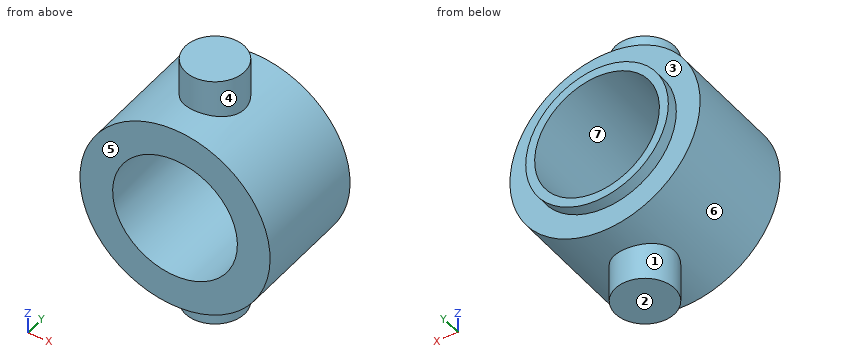
from build123d import *

# Parameters (mm, degrees)
SKETCH1_R           = 8
SKETCH1_R_2         = 5.25
BOSS_EXTRUDE1_DEPTH = 5
SKETCH2_R           = 6
SKETCH2_R_2         = 5.25
BOSS_EXTRUDE2_DEPTH = 1
SKETCH3_R           = 2.5
BOSS_EXTRUDE3_DEPTH = 5


with BuildPart() as part:
    # Sketch1 → Boss-Extrude1 (new, symmetric)
    with BuildSketch(Plane(origin=(0, 0, 0), x_dir=(1, 0, 0), z_dir=(0, 1, 0))):
        with Locations(Location((0, 0, 0), (0, 0, 270))):
            Circle(SKETCH1_R)
        with Locations(Location((0, 0, 0), (0, 0, 270))):
            Circle(SKETCH1_R_2, mode=Mode.SUBTRACT)
    extrude(amount=BOSS_EXTRUDE1_DEPTH, both=True)

    # Sketch2 → Boss-Extrude2 (add, symmetric)
    with BuildSketch(Plane(origin=(0, 5, 0), x_dir=(1, 0, 0), z_dir=(0, 1, 0))):
        with Locations(Location((0, 0, 0), (0, 0, 270))):
            Circle(SKETCH2_R)
        with Locations(Location((0, 0, 0), (0, 0, 270))):
            Circle(SKETCH2_R_2, mode=Mode.SUBTRACT)
    extrude(amount=BOSS_EXTRUDE2_DEPTH, both=True)

    # Sketch3 → Boss-Extrude3 (add)
    with BuildSketch(Plane.XY.offset(6)):
        with Locations(Location((0, 0, 0), (0, 0, 180))):
            Circle(SKETCH3_R)
    boss_extrude3 = extrude(amount=BOSS_EXTRUDE3_DEPTH)

    # Mirror1: Boss-Extrude3 across plane
    add(boss_extrude3.mirror(Plane.XY))


solid = part.part
Can you work these out from the model? Positions are in its coordinate system, mm. Face numbers are marked on the shaded views. A direction names the side the tool comes from. Coordinates: 2 decimals unless noted, no trailing zeros. Write each loop counter-clockwise with the first axis right and the second up, starting at its lowest first coordinate (ties: lowest second). Pieces come first, ordered by that corner, then holes. Notation, with made-up numbers: (-14, 14) -> (6, 14) arc R24 ccw to (6, 37) -> close; hole circle Ø5 at (-24.75, 81). An arc over 180 degrees is marked (long way). Write item = value, one per line.
(1) Imagine slicing it at D-D (x = 2.25). Please give me the cut outline in (y, z).
Verdict:
outline = (-5, -7.68) -> (-1.09, -7.68) -> (-1.09, -11) -> (1.09, -11) -> (1.09, -7.68) -> (5, -7.68) -> (5, -5.56) -> (6, -5.56) -> (6, -4.74) -> (-5, -4.74) -> close; (-5, 4.74) -> (6, 4.74) -> (6, 5.56) -> (5, 5.56) -> (5, 7.68) -> (1.09, 7.68) -> (1.09, 11) -> (-1.09, 11) -> (-1.09, 7.68) -> (-5, 7.68) -> close
(2) If I drill on probe 1 along X at (y, z) = (3.25, 0); probe 2 along Y at (x, z) = (-5, 4); probe 3 along Z at (x, y) = (-3, -4), over which ranges is the centre line in solid material (lowest first)?
Verdict:
probe_1 = -8 to -5.25, 5.25 to 8
probe_2 = -5 to 5
probe_3 = -7.42 to -4.31, 4.31 to 7.42
(3) Imagine slicing it at C-C (y = 0). Please give me the cut outline in (x, z).
Verdict:
outline = (-2.5, -11) -> (2.5, -11) -> (2.5, -7.6) arc R8 ccw to (2.5, 7.6) -> (2.5, 11) -> (-2.5, 11) -> (-2.5, 7.6) arc R8 ccw to (-2.5, -7.6) -> close; hole circle Ø10.5 at (0, 0)
(4) For pin 1 (2 mm diameter, centred on y = 0, z = 2, fed in from -X); pin 2 (5 mm diameter, centred on y = 3, z = -4, fed in from +X); pin 3 (4 mm diameter, centred on y = 1, z = -7.5, fed in from +X), each with a flat end and sliding along its axis, tell me the tip position at first contact or that it passes through.
Verdict:
pin_1 = -7.94
pin_2 = 7.86
pin_3 = 5.81
(5) Imagine slicing it at B-B (x = 0). Please give me the cut outline in (y, z), and give its area (3 significant figures).
Verdict:
outline = (-5, -8) -> (-2.5, -8) -> (-2.5, -11) -> (2.5, -11) -> (2.5, -8) -> (5, -8) -> (5, -6) -> (6, -6) -> (6, -5.25) -> (-5, -5.25) -> close; (-5, 5.25) -> (6, 5.25) -> (6, 6) -> (5, 6) -> (5, 8) -> (2.5, 8) -> (2.5, 11) -> (-2.5, 11) -> (-2.5, 8) -> (-5, 8) -> close
area = 86.5 mm^2
(6) On a 3-axis mill with a long thin cutter (end or side, diameter ignored), from which of +Z, -Z, +X, -X, +Y, -Y can I reach the whole of each face in a straight line? I mean the marked faces 1, 2, 3 and 4. Say none if no direction works.
Verdict:
face_1 = -Z
face_2 = -Z, +X, -X, +Y, -Y
face_3 = +Y
face_4 = +Z
(7) Thinking about a two-plate mould opening in Z: for the marked faces 5, 6 and 7, which applies, +Z half, -Z half, draft (parallel to the pull), parting line (faces both ways), or undercut?
Verdict:
face_5 = draft
face_6 = parting line
face_7 = undercut
(8) Imagine slicing it at A-A (z = 0). Please give me the cut outline in (x, y), and give its area (3 significant figures).
Verdict:
outline = (-8, -5) -> (-5.25, -5) -> (-5.25, 6) -> (-6, 6) -> (-6, 5) -> (-8, 5) -> close; (5.25, -5) -> (8, -5) -> (8, 5) -> (6, 5) -> (6, 6) -> (5.25, 6) -> close
area = 56.5 mm^2
